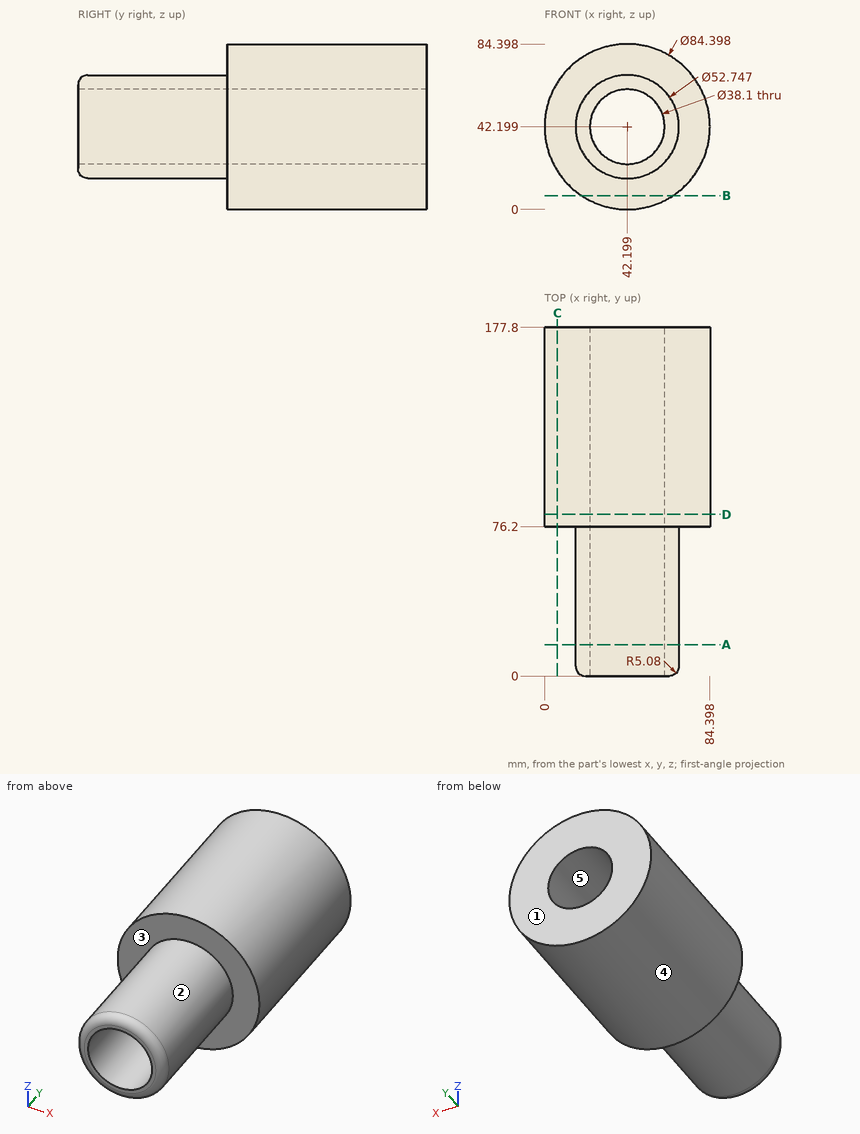
Geometry check sheet. Reference: drawing and pictorial views, mm from the part's lowest x, y, z. A direction names the side the tool comes from. Coordinates: 2 decimals unless noted, no trailing zeros. Order: outer loops, then holes, each group sorted by start corner. A loop starts at its lowest first (then second) coordinate and runs counter-clockwise, first axis right, second up.
Item 1: Scan lines: line 1 along Z through (x, y) = (42, 142); line 2 along Y through (x, z) = (67.5, 75.5); line 3 along Z through (x, y) = (39.5, 138.5). Record each from-to range of solid material in increasing order.
Item 2: Section check A-A (y = 16). Enter the section's corners in (x, z).
Item 3: Tool access check on the marked faces 1 and 2. Record the directions out of +Z, -Z, +X, -X, +Y, -Y that give a thin tool (end or side, any length) a straight path to the whole face; none if there is none.
Item 4: Section check C-C (x = 6.5). Enter the section's corners in (y, z), plus the area to 3 significant figures.
Item 5: Section check B-B (z = 7). Enter the section's corners in (x, y) (1 decimal).
Item 6: Mould release check, pull along Z, two halves, no side actions. Record for the marked faces 3, 4 and 5: released by +Z, released by -Z, zero draft, split by the parting line, or undercut.
Item 7: Section check D-D (y = 82.5). Enter the section's corners in (x, z), plus the area to 3 significant figures.
Item 8: Depth check by flat-ended pin: pin 1 (4 mm diameter, centred on x = 60.5, z = 41, fed in from +Y); pin 2 (1 mm diameter, centred on x = 13, y = 156, fed in from +Z); pin 3 (1 mm diameter, centred on x = 47, z = 20.5, fed in from -Y); pin 4 (8 mm diameter, centred on x = 18, y = 29, fed in from +Z). Enter the tip coordinate at first touch or a pass-through.
Check sheet entries:
1. line 1: z = 0 to 23.15, 61.25 to 84.4
1. line 2: y = 76.2 to 177.8
1. line 3: z = 0.09 to 23.34, 61.06 to 84.31
2. outline: circle Ø52.75 at (42.2, 42.2); hole circle Ø38.1 at (42.2, 42.2)
3. face 1: +Z, -Z, +X, -X, +Y
3. face 2: -Y
4. outline: (76.2, 19.7) - (177.8, 19.7) - (177.8, 64.7) - (76.2, 64.7) - close
4. area: 4,570 mm2
5. outline: (18.9, 76.2) - (65.5, 76.2) - (65.5, 177.8) - (18.9, 177.8) - close
6. face 3: zero draft
6. face 4: split by the parting line
6. face 5: undercut
7. outline: circle Ø84.4 at (42.2, 42.2); hole circle Ø38.1 at (42.2, 42.2)
7. area: 4,450 mm2
8. pin 1: stops at y = 177.8
8. pin 2: stops at z = 73.14
8. pin 3: stops at y = 0.02
8. pin 4: stops at z = 59.16
